Work out the finished part from the listing and answer in its coordinate system (mm). A direction names the side the tool comes from. Coordinates: 2 decimals unless noted, no trailing zeros. Write each loop counter-clockwise with the first axis right and the second up, starting at its lowest first coordinate (ties: lowest second). Pieces come first, ordered by that corner, then holes. Notation, with made-up numbers: (16, 16) - (66, 16) arc R26 ccw to (66, 43) - close; hole circle Ø7 at (12.25, 49). An arc over 180 degrees is marked (long way). Use a Markdown table: item, result. Add a question column.
(1) The part is cut by section B-B, the plane y = 307.5. Give the vertices of the cut face in (x, z), then the cut area to 3 significant figures.
(2) The part is cut by section A-A, the plane x = 443.5. Give the vertices of the cut face in (y, z).
(3) A tool of negligible diameter and unlimited length cuts with its end or side. For faces 4 (the face through (296, 307, -226)), 5 (the face through (296, 18, -787)), 6 (the face through (296, 582, -367)), from which of +Z, -Z, +X, -X, +Y, -Y can it reach the whole face along a straight path? Write none if from no direction.
(4) For a pull along X with two mould halves and no side action, classify faces 1 (the face through (296, 307, -244)), 2 (the face through (17, 279, 0)), 3 (the face through (0, 313, -409)) as released by +X, released by -X, zero draft, split by the parting line, or undercut.
(5) Given pin 1 Ø2 at (x, y) = (271, 430.5) entering from +Z; pin 2 Ø1.5 at (y, z) = (142, -574) entering from -X; pin 3 Ø2 at (x, z) = (90.5, -429) entering from -Y, each flat-ended and moving along its own axis, determine where each tip first touches the part or whether it passes through.
(6) Find the intervals of material crossed by line 1 (Z direction, x = 355.5, y = 535.5); line 2 (X direction, y = 374.5, z = -685); line 3 (Y direction, x = 546.5, z = -433), in increasing order. Write a range as from..to.
(7) The part is cut by section C-C, the plane z = -212.5. Give the vertices of the cut face in (x, y).
(8) The part is cut by section D-D, the plane x = -57. Give the vertices of the cut face in (y, z), then the cut area to 3 significant figures.
from build123d import *

# Parameters (mm, degrees)
F0_W     = 564
F0_H     = 564
F1_DEPTH = 830
F2_W     = 282
F2_H     = 724
F3_DEPTH = 244
F4_W     = 564
F4_H     = 564
F5_DEPTH = 18
F6_W     = 564
F6_H     = 18
F7_DEPTH = 558


with BuildPart() as f1:
    # F0 (on Top) → F1 (new body)
    with BuildSketch(Plane.XY):
        Polygon((-130, 0), (0, 0), (600, 0), (600, 600), (0, 600), (0, 18), (-130, 18), align=None)
        with Locations((300, 300)):
            Rectangle(F0_W, F0_H, mode=Mode.SUBTRACT)
    extrude(amount=-F1_DEPTH)

    # F2 (on face) → F3 (cut)
    with BuildSketch(Plane.XZ):
        with Locations((159, -400)):
            Rectangle(F2_W, F2_H)
        with Locations((441, -400)):
            Rectangle(F2_W, F2_H)
    extrude(amount=-F3_DEPTH, mode=Mode.SUBTRACT)

    # F4 (on face) → F5 (join)
    with BuildSketch(Plane(origin=(0, 0, -830), x_dir=(1, 0, 0), z_dir=(0, 0, -1))):
        with Locations((300, -300)):
            Rectangle(F4_W, F4_H)
    extrude(amount=-F5_DEPTH)

    # F6 (on face) → F7 (join)
    with BuildSketch(Plane.XZ.offset(-582)):
        with Locations((300, -235)):
            Rectangle(F6_W, F6_H)
        with Locations((300, -503)):
            Rectangle(F6_W, F6_H)
    extrude(amount=F7_DEPTH)


solid = f1.part
Model answer:
| question | item | result |
|---|---|---|
| 1 | outline | (0, -830) - (600, -830) - (600, 0) - (582, 0) - (582, -226) - (18, -226) - (18, 0) - (0, 0) - close; hole (18, -812) - (582, -812) - (582, -512) - (18, -512) - close; hole (18, -494) - (582, -494) - (582, -244) - (18, -244) - close |
| 1 | area | 60,300 mm^2 |
| 2 | outline | (0, -830) - (600, -830) - (600, 0) - (582, 0) - (582, -226) - (24, -226) - (24, -244) - (582, -244) - (582, -494) - (24, -494) - (24, -512) - (582, -512) - (582, -812) - (18, -812) - (18, -762) - (0, -762) - close; (0, -38) - (18, -38) - (18, 0) - (0, 0) - close |
| 3 | face 4 | +Z, -Y |
| 3 | face 5 | +Z |
| 3 | face 6 | -Y |
| 4 | face 1 | undercut |
| 4 | face 2 | zero draft |
| 4 | face 3 | released by -X |
| 5 | pin 1 | z = -226 |
| 5 | pin 2 | x = 0 |
| 5 | pin 3 | y = 582 |
| 6 | line 1 | -830..-812, -512..-494, -244..-226 |
| 6 | line 2 | 0..18, 582..600 |
| 6 | line 3 | 582..600 |
| 7 | outline | (-130, 0) - (18, 0) - (18, 582) - (582, 582) - (582, 0) - (600, 0) - (600, 600) - (0, 600) - (0, 18) - (-130, 18) - close |
| 8 | outline | (0, -830) - (18, -830) - (18, 0) - (0, 0) - close |
| 8 | area | 14,900 mm^2 |
